Input: part model. Units: mm. Frame: model coordinates. Face numbers are marked on the shaded views. A direction names the side the tool comes from. Coordinates: 2 decimals unless noted, no trailing zeros. Loops run counter-clockwise (first coordinate to the right, second up) from the corner with the lowest first, then second, coordinate; pieces in that order, holes last. Notation, with made-up numbers: (-33.5, 79) - (23.5, 79) arc R10 cw to (23.5, 88) - close; hole circle Ø2 at (87.25, -4). An arc over 180 degrees is marked (long way). Use one line per item in the form item = value.
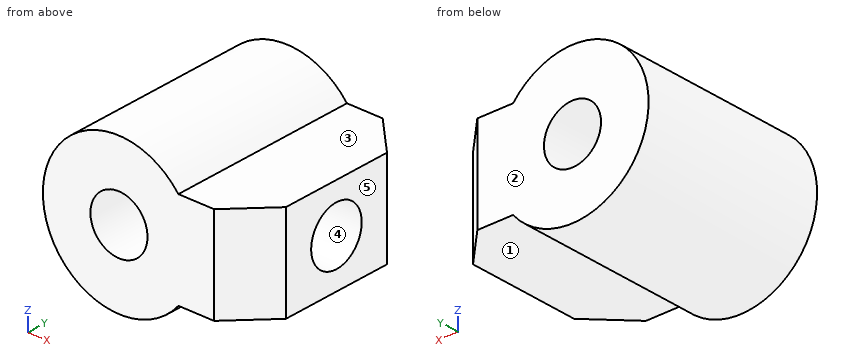
Autodesk Inventor part; units mm, degrees
ref_plane "XY Plane" through (0, 0, 0) normal (0, 0, 1) x (1, 0, 0)
sketch "Sketch1" plane through (0, 0, 0) normal (0, 1, 0) x (-1, 0, 0)
  circle A0 centre (0, 0) radius 4
  circle A1 centre (0, 0) radius 1.5
  dimension "d0" = 8
  dimension "d1" = 3
extrude "Extrusion1" add sketch "Sketch1" along normal blind 10
ref_plane "Work Plane1" through (4, 0, 0) normal (1, 0, 0) x (0, 1, 0)
sketch "Sketch2" plane through (4, 0, 0) normal (1, 0, 0) x (0, 1, 0)
  line L0 (0, -4) -> (10, -4)
  line L1 (10, -4) -> (10, 4)
  line L2 (0, -4) -> (10, -4)
  line L3 (10, -4) -> (10, 4)
  line L4 (10, 4) -> (0, 4)
  line L5 (0, 4) -> (0, -4)
  line L6 (0, 0) -> (0, 2.5)
  line L7 (0, -4) -> (0, 4)
  line L8 (0, 2.5) -> (0, -2.5)
  line L9 (0, -2.5) -> (10, -2.5)
  line L10 (0, 2.5) -> (10, 2.5)
  dimension "d5" = 2.5
  dimension "d6" = 5
extrude "Extrusion2" add sketch "Sketch2" along normal blind 3 and the other way blind 2.5 contours L5 L10 L1 L9
sketch "Sketch3" plane through (7, 0, 0) normal (1, 0, 0) x (0, 0, -1)
  line L0 (0, 0) -> (0, 10)
  line L1 (4, 10) -> (-4, 10)
  circle A0 centre (0, 5) radius 1.5
  point P0 (2.5, 10)
  point P1 (-2.5, 10)
  dimension "d11" = 3
extrude "Extrusion3" cut sketch "Sketch3" against normal blind 5
ref_plane "Work Plane2" through (0, 5, 0) normal (0, 1, 0) x (-1, 0, 0)
chamfer "Chamfer2" distance 2 angle 45 2 edges at (7, 10, 0) (7, 0, 0)
properties part number "joint"
Q1. Cut plane D-D, the plane x = 6.5. Return loops of the section in (y, z).
Check values:
outline = (1.5, -2.5) - (8.5, -2.5) - (8.5, 2.5) - (1.5, 2.5) - close; hole circle Ø3 at (5, 0)
Q2. First-contact query: P1, Ø1.2, axis at x = 4.5, y = 5.5, coming from the +Z side; P2, Ø2.5, axis at y = 5, z = 0, coming from the +X side; P3, Ø2, axis at y = 8.5, z = 3, coming from the -X side. Flat tips, straight axial feed; report the tip coordinate or a pass-through.
Check values:
P1 = 2.5
P2 = 2
P3 = -3.46
Q3. Cut plane A-A, the plane x = 0. Return loops of the section in (y, z), then the cut area to 3 significant figures.
Check values:
outline = (0, -4) - (10, -4) - (10, -1.5) - (0, -1.5) - close; (0, 1.5) - (10, 1.5) - (10, 4) - (0, 4) - close
area = 50.0 mm²
Q4. Pull-direction query (Z, two-part tool) for the marked faces 3, 4 and 5; classes: pulls with the +Z half, pulls with the -Z half, needs draft (parallel to the pull), parting line crosses it, or undercut.
Check values:
face_3 = pulls with the +Z half
face_4 = undercut
face_5 = needs draft
Q5. Cut plane C-C, the plane y = 8.5. Return loops of the section in (x, z), then the cut area to 3 significant figures.
Check values:
outline = (3.12, -2.5) - (6.5, -2.5) - (6.5, 2.5) - (3.12, 2.5) arc R4 ccw (long way) to start; hole circle Ø3 at (0, 0)
area = 57.1 mm²
Q6. Cut plane B-B, the plane z = 0. Return loops of the section in (x, y), then the cut area to 3 significant figures.
Check values:
outline = (-4, 0) - (-1.5, 0) - (-1.5, 10) - (-4, 10) - close; (1.5, 0) - (5, 0) - (7, 2) - (7, 3.5) - (2, 3.5) - (2, 6.5) - (7, 6.5) - (7, 8) - (5, 10) - (1.5, 10) - close
area = 61.0 mm²
Q7. Set-up query: the marked faces 1 and 2. Return all of +Z, -Z, +X, -X, +Y, -Y with unobstructed straight access to the full face (end or side cutting, diameter ignored); none if empty.
Check values:
face_1 = -Z, +X, +Y, -Y
face_2 = +Z, -Z, +X, -X, +Y
Q8. Ray query, line 1 along Z through (x, y) = (4.7, 5); line 2 along Z through (x, y) = (0, 6); line 3 along Y through (x, z) = (4.5, 1). Return the intervals inside material, ascending. Write a range as [from, to].
Check values:
line_1 = [-2.5, -1.5], [1.5, 2.5]
line_2 = [-4, -1.5], [1.5, 4]
line_3 = [0, 3.88], [6.12, 10]
